from build123d import *

# Parameters (mm, degrees)
F0_R     = 7.25
F1_DEPTH = 12.7


with BuildPart() as f1:
    # F0 (on Right) → F1 (new body)
    with BuildSketch(Plane.YZ):
        with BuildLine():
            ThreePointArc((-21.75, -7.25), (-17.503048, -17.503048), (-7.25, -21.75))
            Line((-7.25, -21.75), (7.25, -21.75))
            ThreePointArc((7.25, -21.75), (17.503048, -17.503048), (21.75, -7.25))
            Line((21.75, -7.25), (21.75, 92.070023))
            ThreePointArc((21.75, 92.070023), (0, 88.9), (-21.75, 92.070023))
            Line((-21.75, 92.070023), (-21.75, -7.25))
        make_face()
        Circle(F0_R, mode=Mode.SUBTRACT)
    extrude(amount=F1_DEPTH)


solid = f1.part
Can you work these out from the model? Positions are in its coordinate system, mm. Round coordinates to 2 decimals unless told otherwise and drop trailing zeros. Write each loop counter-clockwise with the first axis right and the second up, starting at its lowest first coordinate (ties: lowest second). Pieces come first, ordered by that corner, then holes. Notation, with made-up numbers: (-39, 34.25) - (-25, 34.25) arc R21 cw to (-25, 50.25) - close; hole circle Ø1 at (13.5, -7). An arc over 180 degrees is marked (long way). Write each question's results on one line, items separated by ' | '. Start each with the question number.
1) Suppose I cut it at A-A (y = 0). List the corners of the cut face in (x, z) for me, and give its area (3 significant figures).
2) Suppose I cut it at D-D (y = 11.5). List the corners of the cut face in (x, z) for me, and give its area (3 significant figures).
3) We'd pull the mould along Y, two halves only. Please class faces 1 (the cylindrical face through (6.3, 0.3, 88.9)), 2 (the flat face through (6, -21.75, 43)), 3 (the flat face through (0, 0, 36)), 4 (the flat face through (6, 21.75, 42)): released by +Y, released by -Y, zero draft, split by the parting line, or undercut.
4) Suppose I cut it at C-C (x = 6.5). List the corners of the cut face in (y, z) for me, and give its area (3 significant figures).
5) Please list where these lines run through material, in increasing order: line 1 (Z direction, x = 6.75, y = 0); line 2 (Z direction, x = 7.75, y = -3); line 3 (Y direction, x = 5.75, z = 2).
6) Suppose I cut it at B-B (z = 0). List the corners of the cut face in (x, y) for me, and give its area (3 significant figures).
Here are the results:
1) outline: (0, -21.75) - (12.7, -21.75) - (12.7, -7.25) - (0, -7.25) - close; (0, 7.25) - (12.7, 7.25) - (12.7, 88.9) - (0, 88.9) - close | area: 1,220 mm2
2) outline: (0, -21.11) - (12.7, -21.11) - (12.7, 89.77) - (0, 89.77) - close | area: 1,410 mm2
3) face 1: undercut | face 2: released by -Y | face 3: zero draft | face 4: released by +Y
4) outline: (-21.75, -7.25) arc R14.5 ccw to (-7.25, -21.75) - (7.25, -21.75) arc R14.5 ccw to (21.75, -7.25) - (21.75, 92.07) arc R76.2 cw to (-21.75, 92.07) - close; hole circle Ø14.5 at (0, 0) | area: 4,600 mm2
5) line 1: z = -21.75 to -7.25, 7.25 to 88.9 | line 2: z = -21.75 to -6.6, 6.6 to 88.96 | line 3: y = -21.75 to -6.97, 6.97 to 21.75
6) outline: (0, -21.75) - (12.7, -21.75) - (12.7, -7.25) - (0, -7.25) - close; (0, 7.25) - (12.7, 7.25) - (12.7, 21.75) - (0, 21.75) - close | area: 368 mm2
